Part model, mm, in its own coordinate system. Face numbers are marked on the shaded views. Coordinates: 2 decimals unless noted, no trailing zeros. Loops run counter-clockwise (first coordinate to the right, second up) from the corner with the lowest first, then second, coordinate; pieces in that order, holes last. Notation, with made-up numbers: (6.25, 82.25) - (65.25, 82.25) arc R16 cw to (65.25, 112.25) - close; hole circle Ø9 at (66.25, -10). An arc over 180 degrees is marked (long way). One line per question, with ' | ' between items. Start each with the question number.
from build123d import *

# Parameters (mm, degrees)
SKETCH1_W           = 120
SKETCH1_H           = 205
BOSS_EXTRUDE1_DEPTH = 10
BOSS_EXTRUDE2_DEPTH = 5
SKETCH3_W           = 20.5
SKETCH3_H           = 3.2
CUT_EXTRUDE1_DEPTH  = 10
SKETCH4_W           = 20
SKETCH4_H           = 3
BOSS_EXTRUDE3_DEPTH = 10
SKETCH5_W           = 5.2
SKETCH5_H           = 3.2
CUT_EXTRUDE2_DEPTH  = 5


with BuildPart() as part:
    # Sketch1 → Boss-Extrude1 (new body)
    with BuildSketch(Plane(origin=(0, 0, 0), x_dir=(0, 1, 0), z_dir=(0, 0, 1))):
        Rectangle(SKETCH1_W, SKETCH1_H)
    extrude(amount=BOSS_EXTRUDE1_DEPTH)

    # Sketch2 → Boss-Extrude2 (add)
    with BuildSketch(Plane.XY.offset(10)):
        Polygon((-97.5, -55), (97.5, -55), (97.5, 60), (102.5, 60), (102.5, -60), (-102.5, -60), (-102.5, 10), (-97.5, 10), align=None)
    extrude(amount=BOSS_EXTRUDE2_DEPTH)

    # Sketch3 → Cut-Extrude1 (cut)
    with BuildSketch(Plane(origin=(-102.5, 0, 0), x_dir=(0, -1, 0), z_dir=(-1, 0, 0))):
        with Locations((-30, 5)):
            Rectangle(SKETCH3_W, SKETCH3_H)
    extrude(amount=-CUT_EXTRUDE1_DEPTH, mode=Mode.SUBTRACT)

    # Sketch4 → Boss-Extrude3 (add)
    with BuildSketch(Plane(origin=(0, 60, 0), x_dir=(-1, 0, 0), z_dir=(0, 1, 0))):
        with Locations((70, 5)):
            Rectangle(SKETCH4_W, SKETCH4_H)
        with Locations((-70, 5)):
            Rectangle(SKETCH4_W, SKETCH4_H)
    extrude(amount=BOSS_EXTRUDE3_DEPTH)

    # Sketch5 → Cut-Extrude2 (cut)
    with BuildSketch(Plane.XZ.offset(60)):
        with Locations((15, 1.6)):
            Rectangle(SKETCH5_W, SKETCH5_H)
        with Locations((-15, 1.6)):
            Rectangle(SKETCH5_W, SKETCH5_H)
    extrude(amount=-CUT_EXTRUDE2_DEPTH, mode=Mode.SUBTRACT)


solid = part.part
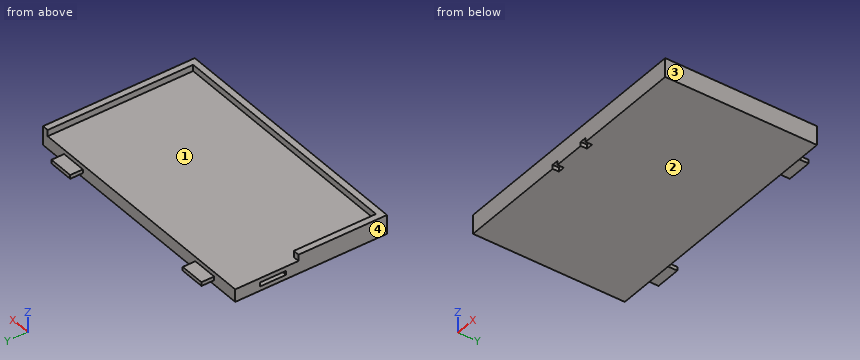
1) Wall check: line 1 along X through (y, z) = (4, 12.75); line 2 along Z through (x, y) = (35, -24); line 3 along X through (y, z) = (28.5, 3.5). Give the ranges that are in metal, low to high. Write a range as [from, to].
2) Band-saw the part on B-B on z = 13. List the corners of the cut face in (x, y).
3) Band-saw the part on C-C on y = -33. List the corners of the cut face in (x, z), then the cut area to 3 significant figures.
4) Band-saw the part on A-A on x = 43. List the corners of the cut face in (y, z), then the cut area to 4 significant figures.
5) Pin check, flat tips, straight feed: pin 1 Ø5.5 at (x, z) = (-47.5, 13.5) entering from +Y; pin 2 Ø3.5 at (y, z) = (67, 4.5) entering from +X; pin 3 Ø8 at (x, y) = (-73, 65) entering from +Z. Stop position of each tip, or through.
6) Mould opens along X. For the marked faces 1, 2, 3 and 4 say: +X half, -X half, draft (parallel to the pull), parting line (faces both ways), or undercut.
7) Band-saw the part on D-D on y = 28.5. List the corners of the cut face in (x, z).
Values found:
1) line 1: [-102.5, -97.5], [97.5, 102.5] | line 2: [0, 10] | line 3: [-92.5, 102.5]
2) outline: (-102.5, -60) - (102.5, -60) - (102.5, 60) - (97.5, 60) - (97.5, -55) - (-97.5, -55) - (-97.5, 10) - (-102.5, 10) - close
3) outline: (-102.5, 0) - (102.5, 0) - (102.5, 15) - (97.5, 15) - (97.5, 10) - (-97.5, 10) - (-97.5, 15) - (-102.5, 15) - close | area: 2,100 mm²
4) outline: (-60, 0) - (60, 0) - (60, 10) - (-55, 10) - (-55, 15) - (-60, 15) - close | area: 1,225 mm²
5) pin 1: y = -55 | pin 2: x = 80 | pin 3: z = 6.5
6) face 1: undercut | face 2: draft | face 3: +X half | face 4: -X half
7) outline: (-102.5, 0) - (102.5, 0) - (102.5, 15) - (97.5, 15) - (97.5, 10) - (-102.5, 10) - (-102.5, 6.6) - (-92.5, 6.6) - (-92.5, 3.4) - (-102.5, 3.4) - close
